Here's how the part is built. I have some questions about the finished solid (model axes, mm). A direction names the side the tool comes from. Round coordinates to 2 decimals unless told otherwise and drop trailing zeros. Write each loop counter-clockwise with the first axis right and the second up, starting at its lowest first coordinate (ties: lowest second). Pieces come first, ordered by that corner, then holes. Notation, with made-up numbers: (8, -34.5) -> (19, -34.5) arc R10 cw to (19, -16.5) -> close; hole circle Ø10 at (44.5, 82.5). An arc over 180 degrees is marked (long way). Answer as CSV lines item,"result".
```python
from build123d import *

# Parameters (mm, degrees)
F0_R     = 1.7526
F0_R_2   = 19.05
F1_DEPTH = 3.175
F2_R     = 12.7


with BuildPart() as f1:
    # F0 (on Top) → F1 (new body)
    with BuildSketch(Plane.XY):
        Polygon((-32.74949, -1.7526), (-32.74949, -6.35), (-38.59149, -6.35), (-38.59149, -19.05), (-32.74949, -19.05), (-32.74949, -22.225), (-20, -26.35), (0, -26.35), (20, -26.35), (32.74949, -22.225), (32.74949, -19.05), (38.59149, -19.05), (38.59149, -6.35), (32.74949, -6.35), (32.74949, -1.7526), (29.57449, -1.7526), (29.57449, -3.048), (26.39949, -3.048), (26.39949, -1.7526), (23.22449, -1.7526), (23.22449, 1.7526), (26.39949, 1.7526), (26.39949, 3.048), (29.57449, 3.048), (29.57449, 1.7526), (32.74949, 1.7526), (32.74949, 6.35), (38.59149, 6.35), (38.59149, 19.05), (32.74949, 19.05), (20, 21.5875), (0, 21.5875), (-20, 21.5875), (-32.74949, 19.05), (-38.59149, 19.05), (-38.59149, 6.35), (-32.74949, 6.35), (-32.74949, 1.7526), (-29.57449, 1.7526), (-29.57449, 3.048), (-26.39949, 3.048), (-26.39949, 1.7526), (-23.22449, 1.7526), (-23.22449, -1.7526), (-26.39949, -1.7526), (-26.39949, -3.048), (-29.57449, -3.048), (-29.57449, -1.7526), align=None)
        with Locations((-16, -16)):
            Circle(F0_R, mode=Mode.SUBTRACT)
        with Locations((16, -16)):
            Circle(F0_R, mode=Mode.SUBTRACT)
        with Locations((-16, 16)):
            Circle(F0_R, mode=Mode.SUBTRACT)
        Circle(F0_R_2, mode=Mode.SUBTRACT)
        with Locations((16, 16)):
            Circle(F0_R, mode=Mode.SUBTRACT)
    extrude(amount=F1_DEPTH)

    # F2
    f2_edges = [f1.edges().sort_by_distance(p)[0] for p in [
        (-20, -26.35, 1.5875),
        (20, -26.35, 1.5875),
        (20, 21.5875, 1.5875),
        (-20, 21.5875, 1.5875),
    ]]
    fillet(f2_edges, radius=F2_R)


solid = f1.part
```
1. Suppose I cut it at C-C on x = 15. Count the separate pieces of the cut face and the enclosed holes in it, and give its area (3 significant figures).
Numbers:
separate pieces,"4"
enclosed holes,"0"
area,"59.4 mm^2"
2. If I drill on line 1 (Y direction, x = 0.5, z = 2.05); line 2 (Y direction, x = -16, z = 1.5); line 3 (X direction, y = -17, z = 2), over which ranges is the centre line in solid material (lowest first)?
Numbers:
line 1,"y = -26.35 to -19.04, 19.04 to 21.59"
line 2,"y = -26.35 to -17.75, -14.25 to -10.34, 10.34 to 14.25, 17.75 to 21.59"
line 3,"x = -38.59 to -17.44, -14.56 to -8.6, 8.6 to 14.56, 17.44 to 38.59"
3. On a 3-axis mill with a long thin cutter (end or side, diameter ignored), from which of +Z, -Z, +X, -X, +Y, -Y can I reach the whole of each face in a straight line? I mean faces 4 (the face through (32.749, -21, 2)), 5 (the face through (-36, -19.05, 2)), 6 (the face through (25, -1.753, 2)). Say none if no direction works.
Numbers:
face 4,"+Z, -Z, +X, -Y"
face 5,"+Z, -Z, -X, -Y"
face 6,"+Z, -Z, +X"
4. Suppose I cut it at A-A on y = 0. Please give me the cut outline in (x, z) (3 decimals).
Numbers:
outline,"(-23.224, 0) -> (-19.05, 0) -> (-19.05, 3.175) -> (-23.224, 3.175) -> close; (19.05, 0) -> (23.224, 0) -> (23.224, 3.175) -> (19.05, 3.175) -> close"
5. For pin 1 Ø1 at (y, z) = (3.5, 1.5) entering from -X; pin 2 Ø1 at (y, z) = (-2.5, 1.5) entering from +X; pin 3 Ø1 at (x, z) = (28.5, 1) entering from -Y, each with a flat end and sliding along its axis, tell me the tip position at first contact or that it passes through.
Numbers:
pin 1,"stops at x = -32.75"
pin 2,"stops at x = 32.75"
pin 3,"stops at y = -23.76"
6. If we mould it in two halves opening along X, with no side actions, what happens to faces 1 (the face through (36, -19.05, 2)), 2 (the face through (27.252, -24.004, 1.565)), 3 (the face through (-17.292, -14.816, 1.565))? For each: released by +X, released by -X, zero draft, split by the parting line, or undercut.
Numbers:
face 1,"zero draft"
face 2,"released by +X"
face 3,"undercut"
7. Suppose I cut it at D-D on y = -16. Please give me the cut outline in (x, z) (3 decimals).
Numbers:
outline,"(-38.591, 0) -> (-17.753, 0) -> (-17.753, 3.175) -> (-38.591, 3.175) -> close; (-14.247, 0) -> (-10.339, 0) -> (-10.339, 3.175) -> (-14.247, 3.175) -> close; (10.339, 0) -> (14.247, 0) -> (14.247, 3.175) -> (10.339, 3.175) -> close; (17.753, 0) -> (38.591, 0) -> (38.591, 3.175) -> (17.753, 3.175) -> close"
